The figure shows three views and two pictorial views of one solid part (mm, origin at its lowest corner). Answer the questions. A direction names the side the tool comes from. Coordinates: 2 decimals unless noted, no trailing zeros. Loops run counter-clockwise (first coordinate to the right, second up) from the corner with the lowest first, then second, coordinate; pieces in that order, holes last. Notation, with made-up numbers: M 83,-6 L 118,-6 A20 ccw 118,15 Z; hole C 10.5,77.25 d10. An arc over 180 degrees is marked long. One line per item, written item: value. Start each with the question number.
1. Determine the mould class of the marked faces 4, 5, 6 and 7 for opening direction Z: +Z half, -Z half, draft (parallel to the pull), parting line (faces both ways), or undercut.
2. The part is cut by section B-B (x = 968.5). Write down the section's boundary in (y, z).
3. For the marked faces 1, 2 and 3, determine the directions among +Z, -Z, +X, -X, +Y, -Y from which every point of the face is accessible in a straight line to the end or side of a thin tool.
4. The part is cut by section D-D (z = 274). Write down the section's boundary in (x, y).
5. The part is cut by section A-A (z = 410). Write down the section's boundary in (x, y).
6. Consider probe 1 along X at (y, z) = (26, 547.5); probe 2 along Z at (x, y) = (116, 215.5); probe 3 along X at (y, z) = (171.5, 68). Determine where each line is inside the solid, lowest interval first.
7. A flat-ended cylindrical pin translates along its axis: pin 1 (8 mm diameter, centred on y = 216, z = 127, fed in from +X). Find the tip coordinate at first contact, or state that the pin passes through.
8. The part is cut by section C-C (y = 107.5). Write down the section's boundary in (x, z).
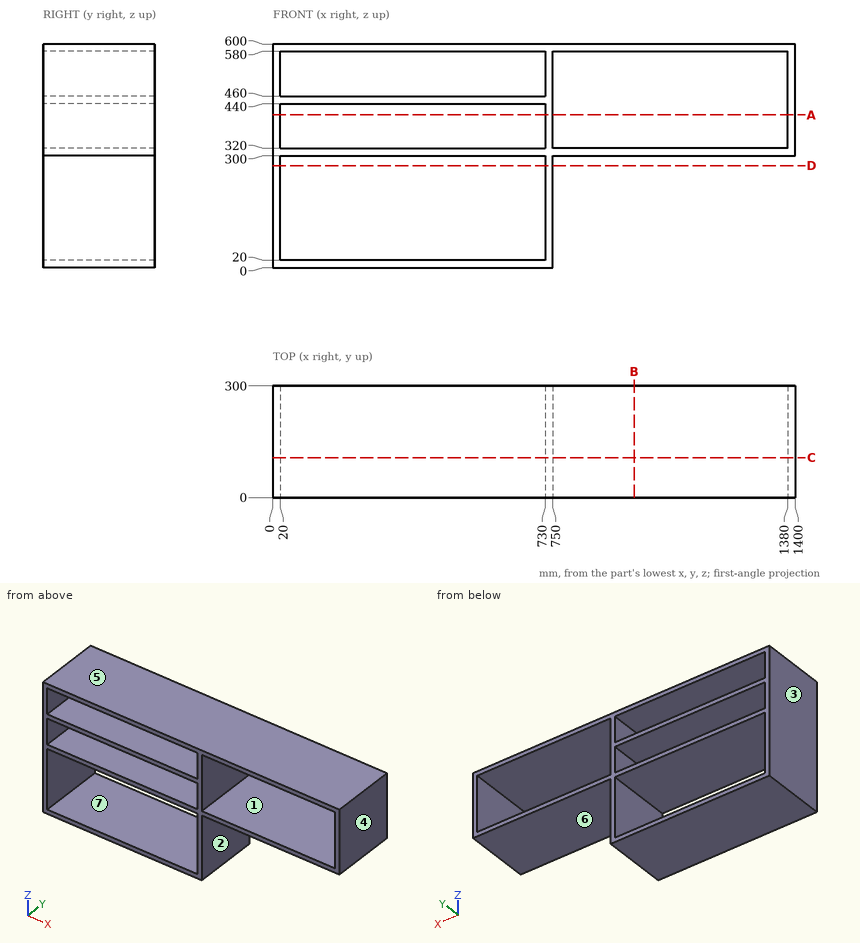
Answer block:
1. face 4: draft
1. face 5: +Z half
1. face 6: -Z half
1. face 7: undercut
2. outline: M 0,300 L 300,300 L 300,320 L 0,320 Z; M 0,580 L 300,580 L 300,600 L 0,600 Z
3. face 1: +Y, -Y
3. face 2: -Z, +X, +Y, -Y
3. face 3: +Z, -Z, -X, +Y, -Y
4. outline: M 0,0 L 20,0 L 20,300 L 0,300 Z; M 730,0 L 750,0 L 750,300 L 730,300 Z
5. outline: M 0,0 L 20,0 L 20,300 L 0,300 Z; M 730,0 L 750,0 L 750,300 L 730,300 Z; M 1380,0 L 1400,0 L 1400,300 L 1380,300 Z
6. probe 1: x = 0 to 20, 730 to 750, 1380 to 1400
6. probe 2: z = 0 to 20, 300 to 320, 440 to 460, 580 to 600
6. probe 3: x = 0 to 20, 730 to 750
7. pin 1: stops at x = 750
8. outline: M 0,0 L 750,0 L 750,300 L 1400,300 L 1400,600 L 0,600 Z; hole M 20,20 L 730,20 L 730,300 L 20,300 Z; hole M 20,320 L 730,320 L 730,440 L 20,440 Z; hole M 20,460 L 730,460 L 730,580 L 20,580 Z; hole M 750,320 L 1380,320 L 1380,580 L 750,580 Z
